Work out the finished part from the listing and answer in its coordinate system (mm). A direction names the side the tool comes from. Coordinates: 2 decimals unless noted, no trailing zeros. Order: outer loops, then holes, each group sorted by start corner. A loop starts at its lowest first (then second) coordinate and runs counter-clockwise, first axis right, second up.
1. Find the intervals of material crossed by probe 1 along X at (y, z) = (13.5, 0); probe 2 along Y at (x, z) = (33, 36.5); probe 3 along Z at (x, y) = (-41, 6.35), in increasing order.
2. A tool of negligible diameter and unlimited length cuts with its end or side. For faces 1 (the flat face through (12.35, 16, 40.37)), 2 (the cylindrical face through (-0.629, 7.867, 44.299)), 3 (the cylindrical face through (27.414, 15.904, -35.37)), 4 (the flat face through (48, 3.2, -3)), from which of +Z, -Z, +X, -X, +Y, -Y can it reach the whole face along a straight path? Write none if from no direction.
3. Determine the mould class of faces 5 (the flat face through (-33.4, 12.7, 21.9)), 6 (the cylindrical face through (-47.27, 1.58, 6.21)), 7 (the flat face through (23.4, 11.2, 26.3)) for opening direction Z: +Z half, -Z half, draft (parallel to the pull), parting line (faces both ways), or undercut.
4. The part is cut by section A-A, the plane y = 6.5. Give the vertices of the cut face in (x, z).
5. The part is cut by section B-B, the plane x = 0. Count the separate pieces of the cut face and the enclosed holes in it, then the cut area to 3 significant figures.
6. Flat-ended cylindrical pins translate along their axes: pin 1 Ø10 at (y, z) = (15.5, 4) entering from +X; pin 2 Ø12 at (x, z) = (4.5, -32) entering from -Y; pin 3 Ø4 at (x, z) = (39.5, 25.5) entering from +Y; pin 4 Ø4.5 at (x, y) = (0, 6.35) entering from -Z. Find the tip coordinate at first contact, or state that the pin passes through.
```python
from build123d import *

# Parameters (mm, degrees)
SKETCH5_R          = 1.6425
CUT_EXTRUDE1_DEPTH = 50.7
SKETCH6_R          = 1.095
CUT_EXTRUDE2_DEPTH = 70.421071799
CIRPATTERN1_COUNT  = 4
CUT_EXTRUDE3_DEPTH = 6.5
CIRPATTERN2_COUNT  = 2
CIRPATTERN2_ANGLE  = 110
CIRPATTERN3_COUNT  = 2
CIRPATTERN3_ANGLE  = 110
CUT_EXTRUDE5_REACH = 13.2


with BuildPart() as part:
    # Sketch2 → Revolve1 (revolve)
    with BuildSketch(Plane.XY, mode=Mode.PRIVATE) as revolve1_sk:
        Polygon((49.7, 12.7), (49.7, 3.2004), (47.675, 3.2004), (47.675, 0), (44.7, 0), (34.75, 9.2), (34.75, 11.2), (39.75, 11.2), (39.75, 19.2), (44.75, 19.2), (44.75, 12.7), align=None)
    revolve(revolve1_sk.sketch.rotate(Axis((0, 0, 0), (0, 1, 0)), 90), axis=Axis((0, 0, 0), (0, 1, 0)))  # turned: the seam where the file's is

    # Sketch5 → Cut-Extrude1 (cut, through all)
    with BuildSketch(Plane.XY):
        with Locations(Location((0, 6.35, 0), (0, 0, 89.999999821))):  # turned: the seam where the file's is
            Circle(SKETCH5_R)
    cut_extrude1 = extrude(amount=-CUT_EXTRUDE1_DEPTH, mode=Mode.SUBTRACT)

    # Sketch6 → Cut-Extrude2 (cut, through all)
    with BuildSketch(Plane(origin=(0, 0, 0), x_dir=(0.809016994, 0, 0.587785252), z_dir=(-0.587785252, 0, 0.809016994))):
        with Locations((0, 15.2)):
            Circle(SKETCH6_R)
    cut_extrude2 = extrude(amount=-CUT_EXTRUDE2_DEPTH, mode=Mode.SUBTRACT)

    # CirPattern1: Cut-Extrude1 ×4 about axis
    cirpattern1_axis = Axis((0, 13.335, 0), (0, -1, 0))
    for i in range(1, CIRPATTERN1_COUNT):
        add(cut_extrude1.rotate(cirpattern1_axis, i * 360 / CIRPATTERN1_COUNT), mode=Mode.SUBTRACT)

    # Sketch7 → Cut-Extrude3 (cut)
    with BuildSketch(Plane(origin=(0, 19.2, 0), x_dir=(-1, 0, 0), z_dir=(0, 1, 0))):
        with BuildLine():
            Line((44.743322047, 0.773066741), (39.744068187, 0.686690568))
            ThreePointArc((39.744068187, 0.686690568), (23.364463779, 32.158425526), (-11.628510956, 38.011054089))
            Line((-11.628510956, 38.011054089), (-13.091216736, 42.792318754))
            ThreePointArc((-13.091216736, 42.792318754), (26.30339004, 36.203510498), (44.743322047, 0.773066741))
        make_face()
    extrude(amount=-CUT_EXTRUDE3_DEPTH, mode=Mode.SUBTRACT)

    # CirPattern2: Cut-Extrude2 ×2 about axis
    cirpattern2_axis = Axis((0, 13.335, 0), (0, -1, 0))
    for i in range(1, CIRPATTERN2_COUNT):
        add(cut_extrude2.rotate(cirpattern2_axis, i * CIRPATTERN2_ANGLE / (CIRPATTERN2_COUNT - 1)), mode=Mode.SUBTRACT)

    # CirPattern3: Cut-Extrude2 ×2 about axis
    cirpattern3_axis = Axis((0, 13.335, 0), (0, 1, 0))
    for i in range(1, CIRPATTERN3_COUNT):
        add(cut_extrude2.rotate(cirpattern3_axis, i * CIRPATTERN3_ANGLE / (CIRPATTERN3_COUNT - 1)), mode=Mode.SUBTRACT)

    # Cut-Extrude5: up to this cone (the profile starts outside it)
    cut_extrude5_end = Plane(origin=(0, 11.2, 0), z_dir=(0, -1, 0)).offset(-30.130652266) * Cone(1.082e-06, 82.647306238, 76.417608788, align=(Align.CENTER, Align.CENTER, Align.MIN), mode=Mode.PRIVATE)
    # Sketch8 → Cut-Extrude5 (cut, up to the surface)
    with BuildSketch(Plane(origin=(0, 11.2, 0), x_dir=(1, 0, 0), z_dir=(0, 1, 0)), mode=Mode.PRIVATE) as cut_extrude5_sk1:
        with BuildLine():
            Line((16.181580734, 30.752543715), (24.24702365, 24.892656429))
            ThreePointArc((24.24702365, 24.892656429), (22.923624839, 31.551662781), (16.181580734, 30.752543715))
        make_face()
    cut_extrude5_tool1 = extrude(cut_extrude5_sk1.sketch, amount=-CUT_EXTRUDE5_REACH, mode=Mode.PRIVATE) - cut_extrude5_end
    add(cut_extrude5_tool1.solids().sort_by_distance((21.35698, 11.2, -29.395361))[0], mode=Mode.SUBTRACT)


solid = part.part
```
Geometry says:
1. probe 1: x = -44.75 to -39.75, 39.75 to 44.75
1. probe 2: y = 3.2 to 12.7
1. probe 3: z = -28.09 to -1.64, 1.64 to 28.09
2. face 1: +Z, -X, +Y
2. face 2: +Z, -Z
2. face 3: +Y
2. face 4: -Y
3. face 5: draft
3. face 6: parting line
3. face 7: undercut
4. outline: (-49.67, -1.64) arc R49.7 ccw to (-1.64, -49.67) - (-1.64, -37.63) arc R37.67 cw to (-37.63, -1.64) - close; (-49.67, 1.64) - (-37.63, 1.64) arc R37.67 cw to (-1.64, 37.63) - (-1.64, 49.67) arc R49.7 ccw to start; (1.64, -49.67) arc R49.7 ccw to (49.67, -1.64) - (37.63, -1.64) arc R37.67 cw to (24.93, -28.24) arc R5 cw to (19.15, -32.44) arc R37.67 cw to (1.64, -37.63) - close; (1.64, 37.63) arc R37.67 cw to (37.63, 1.64) - (49.67, 1.64) arc R49.7 ccw to (1.64, 49.67) - close
5. separate pieces: 4
5. enclosed holes: 0
5. area: 215 mm2
6. pin 1: stops at x = 49.7
6. pin 2: stops at y = 5.9
6. pin 3: stops at y = 12.7
6. pin 4: stops at z = -49.7
